from build123d import *

# Parameters (mm, degrees)
BOSS_EXTRUDE1_DEPTH      = 762
BOSS_EXTRUDE1_DEPTH_BACK = 762
SKETCH6_R                = 4.7625
CUT_EXTRUDE1_DEPTH       = 763.528983056


with BuildPart() as part:
    # Sketch4 → Boss-Extrude1 (new, two sides: drawn at the far end of the back side and taken through both)
    with BuildSketch(Plane(origin=(0, 0, 0), x_dir=(0, 0, -1), z_dir=(1, 0, 0)).offset(-BOSS_EXTRUDE1_DEPTH_BACK)):
        with BuildLine():
            Line((12.7, -11.43), (12.7, 11.43))
            ThreePointArc((12.7, 11.43), (12.328025612, 12.328025612), (11.43, 12.7))
            Line((11.43, 12.7), (-11.43, 12.7))
            ThreePointArc((-11.43, 12.7), (-12.328025612, 12.328025612), (-12.7, 11.43))
            Line((-12.7, 11.43), (-12.7, -11.43))
            ThreePointArc((-12.7, -11.43), (-12.328025612, -12.328025612), (-11.43, -12.7))
            Line((-11.43, -12.7), (11.43, -12.7))
            ThreePointArc((11.43, -12.7), (12.328025612, -12.328025612), (12.7, -11.43))
        make_face()
        with BuildLine():
            Line((11.049, 9.9441), (11.049, -9.9441))
            ThreePointArc((11.049, -9.9441), (10.725382283, -10.725382283), (9.9441, -11.049))
            Line((9.9441, -11.049), (-9.9441, -11.049))
            ThreePointArc((-9.9441, -11.049), (-10.725382283, -10.725382283), (-11.049, -9.9441))
            Line((-11.049, -9.9441), (-11.049, 9.9441))
            ThreePointArc((-11.049, 9.9441), (-10.725382283, 10.725382283), (-9.9441, 11.049))
            Line((-9.9441, 11.049), (9.9441, 11.049))
            ThreePointArc((9.9441, 11.049), (10.725382283, 10.725382283), (11.049, 9.9441))
        make_face(mode=Mode.SUBTRACT)
    extrude(amount=BOSS_EXTRUDE1_DEPTH + BOSS_EXTRUDE1_DEPTH_BACK)

    # Sketch6 → Cut-Extrude1 (cut, through all)
    with BuildSketch(Plane.XY.offset(12.7)):
        with Locations((752.475, 0)):
            Circle(SKETCH6_R)
        with Locations((-752.475, 0)):
            Circle(SKETCH6_R)
    extrude(amount=-CUT_EXTRUDE1_DEPTH, mode=Mode.SUBTRACT)


solid = part.part
Read the model definition and answer for the solid it produces. Units are mm, in the model's axes. Give positions to 0.01 mm unless a question says otherwise; leave off trailing zeros. Loops run counter-clockwise (first coordinate to the right, second up) from the corner with the lowest first, then second, coordinate; pieces in that order, holes last. Notation, with made-up numbers: (68, 87) -> (102, 87) arc R34 cw to (102, 126) -> close; hole circle Ø10 at (65.5, 48.5). An arc over 180 degrees is marked (long way). Answer as CSV lines item,"result".
Item 1: Each of these flat-tipped pins is pushed along its axis until it touches: pin 1 (12.5 mm diameter, centred on x = -752.475, y = 0, fed in from -Z); pin 2 (8 mm diameter, centred on y = 4.5, z = 3, fed in from -X). Where does it stop, or does it pass through?
Returned:
pin 1,"stops at z = -12.7"
pin 2,"passes through"
Item 2: Find section C-C on z = 1. Give the vertices of the cut face in (x, y), plus the area to 3 significant figures.
Returned:
outline,"(-762, -12.7) -> (762, -12.7) -> (762, -11.05) -> (-762, -11.05) -> close; (-762, 11.05) -> (762, 11.05) -> (762, 12.7) -> (-762, 12.7) -> close"
area,"5,030 mm²"
Item 3: Find section A-A on x = 635. Give the vertices of the cut face in (y, z), plus the area to 3 significant figures.
Returned:
outline,"(-12.7, -11.43) arc R1.27 ccw to (-11.43, -12.7) -> (11.43, -12.7) arc R1.27 ccw to (12.7, -11.43) -> (12.7, 11.43) arc R1.27 ccw to (11.43, 12.7) -> (-11.43, 12.7) arc R1.27 ccw to (-12.7, 11.43) -> close; hole (-11.05, -9.94) arc R1.1 ccw to (-9.94, -11.05) -> (9.94, -11.05) arc R1.1 ccw to (11.05, -9.94) -> (11.05, 9.94) arc R1.1 ccw to (9.94, 11.05) -> (-9.94, 11.05) arc R1.1 ccw to (-11.05, 9.94) -> close"
area,"157 mm²"
Item 4: Find section B-B on y = 0. Give the vertices of the cut face in (x, z).
Returned:
outline,"(-762, -12.7) -> (-757.24, -12.7) -> (-757.24, -11.05) -> (-762, -11.05) -> close; (-762, 11.05) -> (-757.24, 11.05) -> (-757.24, 12.7) -> (-762, 12.7) -> close; (-747.71, -12.7) -> (747.71, -12.7) -> (747.71, -11.05) -> (-747.71, -11.05) -> close; (-747.71, 11.05) -> (747.71, 11.05) -> (747.71, 12.7) -> (-747.71, 12.7) -> close; (757.24, -12.7) -> (762, -12.7) -> (762, -11.05) -> (757.24, -11.05) -> close; (757.24, 11.05) -> (762, 11.05) -> (762, 12.7) -> (757.24, 12.7) -> close"
Item 5: Consider line 1 (Z direction, x = -388.5, y = -4); line 2 (Y direction, x = -676, z = 10.75). Determine where each line is inside the solid, lowest interval first. Write a range as [from, to].
Returned:
line 1,"z = [-12.7, -11.05], [11.05, 12.7]"
line 2,"y = [-12.7, -10.7], [10.7, 12.7]"
